The listing builds one solid part. Answer for the finished solid, in the listing's coordinates (mm). A direction names the side the tool comes from. Round coordinates to 2 decimals unless told otherwise and drop trailing zeros. Loops run counter-clockwise (first coordinate to the right, second up) from the corner with the lowest first, then second, coordinate; pieces in that order, holes last. Notation, with made-up numbers: M 66,46 L 124,46 A29 ccw 124,71 Z; hole C -31,77 d4. An arc over 180 degrees is marked long. Put each result on its own line as item: value. Start each with the question number.
(1) Determine the mould class of faces 3 (the face through (29.013, 9.392, -22.363)), 4 (the face through (-1, 5, 0)), 5 (the face through (-14, 16.51, -19)) for opening direction Z: released by +Z, released by -Z, zero draft, split by the parting line, or undercut.
(2) Flat-ended cylindrical pins translate along their axes: P1, Ø12, axis at x = -1.5, z = -12, coming from the +Y side; P2, Ø1.2, axis at x = -15, z = -28, coming from the +Y side; P3, Ø0.7, axis at x = -5, z = -28.5, coming from the +Y side. Find the tip coordinate at first contact, or state that the pin passes through.
(3) Section B-B, the plane y = 4.25 is taken. Determine the outline of the cut face in (x, z) (3 decimals), then the cut area to 3 significant figures.
(4) Section A-A, the plane x = 25.4 is taken. Determine the outline of the cut face in (y, z).
(5) Section C-C, the plane z = -19.05 is taken. Count the separate pieces of the cut face and the enclosed holes in it, then the cut area to 3 significant figures.
(6) Straight lines are drawn through the part: line 1 (X direction, y = 10.25, z = -19.05) (3 decimals); line 2 (X direction, y = 4.75, z = -19.05) (3 decimals); line 3 (Z direction, x = -25.4, y = 12.5). For each, find the intervals that lie inside material, in ascending order.
(7) Which of the six approach directions +Z, -Z, +X, -X, +Y, -Y give full straight-line access (tool end or side, diameter ignored) to faces 1 (the face through (12, 15.24, -19)), 2 (the face through (31, 19.05, -19))?
```python
from build123d import *

# Parameters (mm, degrees)
SKETCH1_W               = 69.85
SKETCH1_H               = 19.05
BOSS_EXTRUDE1_DEPTH     = 38.1
CUT_EXTRUDE1_REACH      = 40.1
F_3_8_CLEARANCE_HOLE1_D = 9.8044
BOSS_EXTRUDE2_DEPTH     = 19.05


with BuildPart() as part:
    # Sketch1 → Boss-Extrude1 (new body)
    with BuildSketch(Plane.XY):
        with Locations((0, 9.525)):
            Rectangle(SKETCH1_W, SKETCH1_H)
    extrude(amount=-BOSS_EXTRUDE1_DEPTH)

    # Sketch2 → Cut-Extrude1 (cut, up to next)
    with BuildSketch(Plane.XY, mode=Mode.PRIVATE) as cut_extrude1_sk1:
        with BuildLine():
            Line((-15.875, 19.05), (0, 19.05))
            Line((0, 19.05), (15.875, 19.05))
            Line((15.875, 19.05), (15.875, 17.78))
            Line((15.875, 17.78), (14.410694861, 17.78))
            Line((14.410694861, 17.78), (14.410694861, 16.51))
            Line((14.410694861, 16.51), (12.946389723, 16.51))
            Line((12.946389723, 16.51), (12.946389723, 15.24))
            Line((12.946389723, 15.24), (11.482084584, 15.24))
            Line((11.482084584, 15.24), (11.482084584, 13.97))
            Line((11.482084584, 13.97), (10.017779445, 13.97))
            Line((10.017779445, 13.97), (10.017779445, 12.7))
            Line((10.017779445, 12.7), (8.553474306, 12.7))
            Line((8.553474306, 12.7), (8.553474306, 11.43))
            Line((8.553474306, 11.43), (7.089169168, 11.43))
            Line((7.089169168, 11.43), (7.089169168, 10.16))
            Line((7.089169168, 10.16), (5.624864029, 10.16))
            Line((5.624864029, 10.16), (5.624864029, 8.89))
            Line((5.624864029, 8.89), (4.16055889, 8.89))
            ThreePointArc((4.16055889, 8.89), (0, 7.337108475), (-4.16055889, 8.89))
            Line((-4.16055889, 8.89), (-5.624864029, 8.89))
            Line((-5.624864029, 8.89), (-5.624864029, 10.16))
            Line((-5.624864029, 10.16), (-7.089169168, 10.16))
            Line((-7.089169168, 10.16), (-7.089169168, 11.43))
            Line((-7.089169168, 11.43), (-8.553474306, 11.43))
            Line((-8.553474306, 11.43), (-8.553474306, 12.7))
            Line((-8.553474306, 12.7), (-10.017779445, 12.7))
            Line((-10.017779445, 12.7), (-10.017779445, 13.97))
            Line((-10.017779445, 13.97), (-11.482084584, 13.97))
            Line((-11.482084584, 13.97), (-11.482084584, 15.24))
            Line((-11.482084584, 15.24), (-12.946389723, 15.24))
            Line((-12.946389723, 15.24), (-12.946389723, 16.51))
            Line((-12.946389723, 16.51), (-14.410694861, 16.51))
            Line((-14.410694861, 16.51), (-14.410694861, 17.78))
            Line((-14.410694861, 17.78), (-15.875, 17.78))
            Line((-15.875, 17.78), (-15.875, 19.05))
        make_face()
    cut_extrude1_tool1 = extrude(cut_extrude1_sk1.sketch, amount=-CUT_EXTRUDE1_REACH, mode=Mode.PRIVATE) & part.part
    add(cut_extrude1_tool1.solids().sort_by_distance((0, 14.620592, 0))[0], mode=Mode.SUBTRACT)

    # 3/8 Clearance Hole1 (through all)
    with Locations(Plane(origin=(0, 19.05, 0), x_dir=(1, 0, 0), z_dir=(0, 1, 0))):
        with Locations((-25.4, 19.05), (25.4, 19.05)):
            Hole(F_3_8_CLEARANCE_HOLE1_D / 2)

    # Sketch7 → Boss-Extrude2 (add)
    with BuildSketch(Plane(origin=(0, 19.05, 0), x_dir=(1, 0, 0), z_dir=(0, 1, 0))):
        Polygon((-34.925, 38.1), (-41.275, 38.1), (-41.275, 0), (-32.371593609, 0), (-32.371593609, 38.1), align=None)
        Polygon((41.275, 0), (32.371593609, 0), (32.371593609, 38.1), (34.925, 38.1), (41.275, 38.1), align=None)
    extrude(amount=-BOSS_EXTRUDE2_DEPTH)


solid = part.part
```
Recorded:
1. face 3: undercut
1. face 4: released by +Z
1. face 5: zero draft
2. P1: stops at y = 11.43
2. P2: stops at y = 17.78
2. P3: stops at y = 8.89
3. outline: M -41.275,-38.1 L 41.275,-38.1 L 41.275,0 L -41.275,0 Z; hole C -25.4,-19.05 d9.804; hole C 25.4,-19.05 d9.804
3. area: 2,990 mm²
4. outline: M 0,-38.1 L 19.05,-38.1 L 19.05,-23.95 L 0,-23.95 Z; M 0,-14.15 L 19.05,-14.15 L 19.05,0 L 0,0 Z
5. separate pieces: 3
5. enclosed holes: 0
5. area: 972 mm²
6. line 1: x = -41.275 to -30.302, -20.498 to -7.089, 7.089 to 20.498, 30.302 to 41.275
6. line 2: x = -41.275 to -30.302, -20.498 to 20.498, 30.302 to 41.275
6. line 3: z = -38.1 to -23.95, -14.15 to 0
7. face 1: +Z, -Z, +Y
7. face 2: +Z, -Z, +X, -X, +Y
